Check sheet for the modelled part. Datum: model origin and axes. Units: mm. A direction names the side the tool comes from. Round coordinates to 2 decimals unless told otherwise and drop trailing zeros. Loops run counter-clockwise (first coordinate to the right, second up) from the corner with the lowest first, then second, coordinate; pieces in that order, holes last. Notation, with made-up numbers: (-8.75, 23.5) -> (1.25, 23.5) arc R25 cw to (1.25, 36.5) -> close; hole circle Ø8 at (-32.5, 12). An arc over 180 degrees is marked (long way). One line per item, written item: value. Start each with the question number.
1. Go/stop test with flat-tipped pins: pin 1 (1 mm diameter, centred on y = -16, z = -38, fed in from +X); pin 2 (1.6 mm diameter, centred on x = -46.5, z = -37.5, fed in from +Y); pin 3 (1.2 mm diameter, centred on y = -19, z = -5.5, fed in from +X). Record where each tip stops, or that it passes through.
2. Cross-section at D-D on z = 0. Record the cut outline in (x, y).
3. Set-up check for faces 1 (the face through (-49.35, -19, 0)), 2 (the face through (55.75, -9, 0)), 3 (the face through (-46, -16, -36.5)): record each of +Z, -Z, +X, -X, +Y, -Y from which the full face is reachable in a straight line by a thin tool's end or side.
4. Cross-section at B-B on x = 24. Record the cut outline in (y, z).
5. Cross-section at A-A on y = -3. Record the cut outline in (x, z), then the cut area to 3 significant figures.
6. Release check for a two-part mould opening along X. For faces 4 (the face through (46, -16, 33.5)), 5 (the face through (-53.469, -8.874, -40.594)), 6 (the face through (53.469, -8.874, 40.594)), 7 (the face through (51.68, -8.63, 38.85)) record: +X half, -X half, draft (parallel to the pull), parting line (faces both ways), or undercut.
7. Material ranges on L1, parallel to X at y = -14.75, z = -4; L2, parallel to Z at x = -22, y = -15.25, recorded low to high.
8. Cross-section at C-C on z = -22.5. Record the cut outline in (x, y), then the cut area to 3 significant figures.
from build123d import *

# Parameters (mm, degrees)
F1_DEPTH  = 20
F2_T      = -2.5
F5_W      = 98.7
F5_H      = 57.5
F6_DEPTH  = 50
F7_W      = 15
F7_H      = 2
F8_DEPTH  = 6
F11_R     = 2
F12_R     = 1.5
F13_DEPTH = 70


with BuildPart() as f1:
    # F0 (on Front) → F1 (new body)
    with BuildSketch(Plane.XZ):
        with BuildLine():
            Line((47.75, 43), (-47.75, 43))
            ThreePointArc((-47.75, 43), (-53.406854, 40.656854), (-55.75, 35))
            Line((-55.75, 35), (-55.75, -35))
            ThreePointArc((-55.75, -35), (-53.406854, -40.656854), (-47.75, -43))
            Line((-47.75, -43), (47.75, -43))
            ThreePointArc((47.75, -43), (53.406854, -40.656854), (55.75, -35))
            Line((55.75, -35), (55.75, 35))
            ThreePointArc((55.75, 35), (53.406854, 40.656854), (47.75, 43))
        make_face()
    extrude(amount=F1_DEPTH)

    # F2
    f2_openings = [f1.faces().sort_by_distance(p)[0] for p in [
        (0, 0, 0),
    ]]
    offset(amount=F2_T, openings=f2_openings)

    # F5 (on Front) → F6 (cut)
    with BuildSketch(Plane.XZ):
        with Locations((0, -0.05)):
            Rectangle(F5_W, F5_H)
    extrude(amount=F6_DEPTH, mode=Mode.SUBTRACT)

    # F7 (on offset) → F8 (join)
    with BuildSketch(Plane.XZ.offset(20)):
        with Locations((45.943302, -37.5)):
            Rectangle(F7_W, F7_H)
        with Locations((-45.943302, -37.5)):
            Rectangle(F7_W, F7_H)
        with Locations((45.908305, 32.5)):
            Rectangle(F7_W, F7_H)
        with Locations((-45.908305, 32.5)):
            Rectangle(F7_W, F7_H)
    extrude(amount=-F8_DEPTH)

    # F11
    f11_edges = [f1.edges().sort_by_distance(p)[0] for p in [
        (0, -20, 43),
        (55.75, -20, 0),
    ]]
    fillet(f11_edges, radius=F11_R)

    # F12 (on Right) → F13 (cut, symmetric)
    with BuildSketch(Plane.YZ):
        with Locations((-3, 0)):
            Circle(F12_R)
    extrude(amount=F13_DEPTH, both=True, mode=Mode.SUBTRACT)


solid = f1.part
Taken from the geometry:
1. pin 1: stops at x = 55.35
1. pin 2: stops at y = -14
1. pin 3: stops at x = 55.71
2. outline: (-55.75, -18) arc R2 ccw to (-53.75, -20) -> (-49.35, -20) -> (-49.35, -17.5) -> (-53.25, -17.5) -> (-53.25, -4.5) -> (-55.75, -4.5) -> close; (-55.75, -1.5) -> (-53.25, -1.5) -> (-53.25, 0) -> (-55.75, 0) -> close; (49.35, -20) -> (53.75, -20) arc R2 ccw to (55.75, -18) -> (55.75, -4.5) -> (53.25, -4.5) -> (53.25, -17.5) -> (49.35, -17.5) -> close; (53.25, -1.5) -> (55.75, -1.5) -> (55.75, 0) -> (53.25, 0) -> close
3. face 1: +Y, -Y
3. face 2: +Z, -Z, +X, +Y, -Y
3. face 3: +Y
4. outline: (-20, -41) arc R2 ccw to (-18, -43) -> (0, -43) -> (0, -40.5) -> (-17.5, -40.5) -> (-17.5, -28.8) -> (-20, -28.8) -> close; (-20, 28.7) -> (-17.5, 28.7) -> (-17.5, 40.5) -> (0, 40.5) -> (0, 43) -> (-18, 43) arc R2 ccw to (-20, 41) -> close
5. outline: (-55.75, -35) arc R8 ccw to (-47.75, -43) -> (47.75, -43) arc R8 ccw to (55.75, -35) -> (55.75, -1.5) -> (53.25, -1.5) -> (53.25, -35) arc R5.5 cw to (47.75, -40.5) -> (-47.75, -40.5) arc R5.5 cw to (-53.25, -35) -> (-53.25, -1.5) -> (-55.75, -1.5) -> close; (-55.75, 1.5) -> (-53.25, 1.5) -> (-53.25, 35) arc R5.5 cw to (-47.75, 40.5) -> (47.75, 40.5) arc R5.5 cw to (53.25, 35) -> (53.25, 1.5) -> (55.75, 1.5) -> (55.75, 35) arc R8 ccw to (47.75, 43) -> (-47.75, 43) arc R8 ccw to (-55.75, 35) -> close
5. area: 919 mm2
6. face 4: undercut
6. face 5: -X half
6. face 6: +X half
6. face 7: undercut
7. L1: x = -55.75 to -53.25, 53.25 to 55.75
7. L2: z = -43 to -40.5, 40.5 to 43
8. outline: (-55.75, -18) arc R2 ccw to (-53.75, -20) -> (-49.35, -20) -> (-49.35, -17.5) -> (-53.25, -17.5) -> (-53.25, 0) -> (-55.75, 0) -> close; (49.35, -20) -> (53.75, -20) arc R2 ccw to (55.75, -18) -> (55.75, 0) -> (53.25, 0) -> (53.25, -17.5) -> (49.35, -17.5) -> close
8. area: 118 mm2
